Build history of the part. All positions in model axes, mm. A direction names the side the tool comes from. Coordinates: 2 decimals unless noted, no trailing zeros. Loops run counter-clockwise (first coordinate to the right, second up) from the corner with the lowest first, then second, coordinate; pieces in that order, holes last.
Item 1: Flat gauge pins, fed straight in: pin 1 (12 mm diameter, centred on x = 20, y = -33.5, fed in from +Z); pin 2 (10 mm diameter, centred on x = 3, y = -27.5, fed in from -Z); pin 3 (1.5 mm diameter, centred on x = 1.5, z = 41.5, fed in from +Y). Where does each tip first touch, or does it go through?
Item 2: Cut at A-A (y = 14). List the corners of the cut face in (x, z).
Item 3: Mould opens along Y. For faces 1 (the face through (-21, 40.5, 43)), 2 (the face through (0, -41, 83)), 3 (the face through (-19, 42.5, 41)) say: released by +Y, released by -Y, zero draft, split by the parting line, or undercut.
Item 4: Drill centre lines: line 1 along Y through (x, z) = (25.5, 10); line 2 along X through (y, z) = (35, 61.5). Where is each one in solid material? Low to high.
Item 5: Cut at B-B (z = 76). List the corners of the cut face in (x, y), and give its area (3 significant figures).
Item 6: 3-axis set-ups, long thin cutter, end or side, ignore diameter. For faces 4 (the face through (25, 35.5, 43)), 5 (the face through (-1, 1, 0)): which of +Z, -Z, +X, -X, +Y, -Y reach the whole face in a straight line?
Item 7: Cut at C-C (x = -3.5). List the corners of the cut face in (y, z).
from build123d import *

# Parameters (mm, degrees)
SKETCH_W        = 85
SKETCH_H        = 85
PAD_DEPTH       = 83
POCKET_DEPTH    = 82
SKETCH002_W     = 33
SKETCH002_H     = 82
POCKET001_DEPTH = 5


with BuildPart() as part:
    # Sketch → Pad (new body)
    with BuildSketch(Plane.XY):
        Rectangle(SKETCH_W, SKETCH_H)
    extrude(amount=PAD_DEPTH)

    # Sketch001 (on DatumPlane) → Pocket (cut)
    with BuildSketch(Plane(origin=(0, 0, 83), x_dir=(1, 0, 0), z_dir=(0, 0, -1))):
        Polygon((-40.5, 40.5), (-40.5, -40.5), (-28, -40.5), (-28, -35.5), (-22, -35.5), (-22, -37.5), (-26, -37.5), (-26, -40.5), (26, -40.5), (26, -37.5), (22, -37.5), (22, -35.5), (28, -35.5), (28, -40.5), (40.5, -40.5), (40.5, 40.5), align=None)
    extrude(amount=POCKET_DEPTH, mode=Mode.SUBTRACT)

    # Sketch002 (on DatumPlane) → Pocket001 (cut)
    with BuildSketch(Plane.XZ.offset(-42.5)):
        with Locations((0, 42)):
            Rectangle(SKETCH002_W, SKETCH002_H)
    extrude(amount=POCKET001_DEPTH, mode=Mode.SUBTRACT)


solid = part.part
Filled sheet:
1. pin 1: stops at z = 1
1. pin 2: stops at z = 0
1. pin 3: stops at y = -40.5
2. outline: (-42.5, 0) - (42.5, 0) - (42.5, 83) - (40.5, 83) - (40.5, 1) - (-40.5, 1) - (-40.5, 83) - (-42.5, 83) - close
3. face 1: undercut
3. face 2: zero draft
3. face 3: released by +Y
4. line 1: y = -42.5 to -40.5, 35.5 to 37.5, 40.5 to 42.5
4. line 2: x = -42.5 to -40.5, 40.5 to 42.5
5. outline: (-42.5, -42.5) - (42.5, -42.5) - (42.5, 42.5) - (16.5, 42.5) - (16.5, 40.5) - (26, 40.5) - (26, 37.5) - (22, 37.5) - (22, 35.5) - (28, 35.5) - (28, 40.5) - (40.5, 40.5) - (40.5, -40.5) - (-40.5, -40.5) - (-40.5, 40.5) - (-28, 40.5) - (-28, 35.5) - (-22, 35.5) - (-22, 37.5) - (-26, 37.5) - (-26, 40.5) - (-16.5, 40.5) - (-16.5, 42.5) - (-42.5, 42.5) - close
5. area: 634 mm2
6. face 4: +Z
6. face 5: -Z, +X, -X, +Y, -Y
7. outline: (-42.5, 0) - (42.5, 0) - (42.5, 1) - (-40.5, 1) - (-40.5, 83) - (-42.5, 83) - close
